The listing builds one solid part. Answer for the finished solid, in the listing's coordinates (mm). A direction names the side the tool comes from. Coordinates: 2 decimals unless noted, no trailing zeros. Loops run counter-clockwise (first coordinate to the right, second up) from the corner with the lowest first, then second, coordinate; pieces in that order, holes last. Notation, with made-up numbers: (39, 23.25) - (64, 23.25) arc R12 ccw to (64, 46.25) - close; hole circle Ø3 at (-9.5, 63). An arc over 180 degrees is marked (long way). Put each result on its own line as item: value.
Autodesk Inventor part; units mm, degrees
ref_plane "YZ Plane" through (0, 0, 0) normal (1, 0, 0) x (0, 1, 0)
ref_plane "XZ Plane" through (0, 0, 0) normal (0, 1, 0) x (-1, 0, 0)
ref_plane "XY Plane" through (0, 0, 0) normal (0, 0, 1) x (1, 0, 0)
sketch "Sketch1" plane through (0, 0, 0) normal (1, 0, 0) x (0, 1, 0)
  line L0 (7, 0.625) -> (0, 0.625)
  line L1 (1, 1.45) -> (1, 3.5)
  line L2 (2, 2.45) -> (2, 1.5)
  line L3 (7, 1.5) -> (7, 0.625)
  line L4 (-1.4, 0) -> (8.4, 0)
  line L5 (1.5, 2.45) -> (2, 2.45)
  line L6 (1, 3.5) -> (1.5, 3.5)
  line L7 (1.5, 3.5) -> (1.5, 2.45)
  line L8 (1, 1.45) -> (0, 1.45)
  line L9 (0, 1.45) -> (0, 0.625)
  line L10 (7, 1.5) -> (2, 1.5)
  point P0 (0, 0)
  dimension "d0" = 7
  dimension "d1" = 0.625
  dimension "d8" = 2.45
  dimension "d10" = 0.5
  dimension "d11" = 0.5
  dimension "d13" = 3.5
  dimension "d16" = 1
  dimension "d31" = 1.45
  dimension "d32" = 1.5
revolve "Revolution1" add sketch "Sketch1" angle 360 about axis through (0, -10, 0) along (0, 1, 0)
sketch "Sketch5" plane through (0, 7, 0) normal (0, 1, 0) x (1, 0, 0)
  circle A0 centre (0, 0) radius 0.75
  dimension "d28" = 1.5
extrude "Extrusion2" cut sketch "Sketch5" against normal blind 3
properties part number "TorsOsc-202511-cell-tower" material "Epoxy Resin"
1) Straight lines are drawn through the part: L1, parallel to X at y = 4.8, z = 0; L2, parallel to Z at x = 2.5, y = 1.25; L3, parallel to X at y = 3.1, z = 0 (3 decimals). For each, find the intervals that lie inside material, in ascending order. Write a range as [from, to].
Found:
L1: x = [-1.5, -0.75], [0.75, 1.5]
L2: z = [-2.45, 2.45]
L3: x = [-1.5, -0.625], [0.625, 1.5]
2) The part is cut by section B-B (z = 0). Give the vertices of the cut face in (x, y) (3 decimals).
Found:
outline: (-3.5, 1) - (-1.45, 1) - (-1.45, 0) - (-0.625, 0) - (-0.625, 4) - (-0.75, 4) - (-0.75, 7) - (-1.5, 7) - (-1.5, 2) - (-2.45, 2) - (-2.45, 1.5) - (-3.5, 1.5) - close; (0.625, 0) - (1.45, 0) - (1.45, 1) - (3.5, 1) - (3.5, 1.5) - (2.45, 1.5) - (2.45, 2) - (1.5, 2) - (1.5, 7) - (0.75, 7) - (0.75, 4) - (0.625, 4) - close
3) Each of these flat-tipped pins is pushed along its axis until it touches: pin 1 (2 mm diameter, centred on x = -1.5, z = 2.5, fed in from -Y); pin 2 (2 mm diameter, centred on x = 0, z = 0, fed in from +Y); pin 3 (1 mm diameter, centred on x = 0, z = 2.5, fed in from +Y); pin 4 (1 mm diameter, centred on x = 0, z = 0, fed in from +Y). Where does it stop, or does it pass through?
Found:
pin 1: stops at y = 1
pin 2: stops at y = 7
pin 3: stops at y = 2
pin 4: passes through
4) The part is cut by section A-A (x = 0). Give the vertices of the cut face in (y, z) (3 decimals), and give its area (4 significant figures).
Found:
outline: (0, -1.45) - (1, -1.45) - (1, -3.5) - (1.5, -3.5) - (1.5, -2.45) - (2, -2.45) - (2, -1.5) - (7, -1.5) - (7, -0.75) - (4, -0.75) - (4, -0.625) - (0, -0.625) - close; (0, 0.625) - (4, 0.625) - (4, 0.75) - (7, 0.75) - (7, 1.5) - (2, 1.5) - (2, 2.45) - (1.5, 2.45) - (1.5, 3.5) - (1, 3.5) - (1, 1.45) - (0, 1.45) - close
area: 14.35 mm^2
5) The part is cut by section D-D (y = 2.5). Give the vertices of the cut face in (x, z) (3 decimals).
Found:
outline: circle Ø3 at (0, 0); hole circle Ø1.25 at (0, 0)
6) The part is cut by section C-C (y = 5). Give the vertices of the cut face in (x, z), and give its area (3 significant figures).
Found:
outline: circle Ø3 at (0, 0); hole circle Ø1.5 at (0, 0)
area: 5.30 mm^2
7) For a pull along X with two mould halves and no side action, classify faces 1 (the face through (-2.4, 1.8, -0.5)), 2 (the face through (0.61, 1.97, -0.14)), 3 (the face through (-2, 2, 0)) as pulls with the +X half, pulls with the -X half, needs draft (parallel to the pull), parting line crosses it, or undercut.
Found:
face 1: parting line crosses it
face 2: undercut
face 3: needs draft
8) For faces 4 (the face through (-2, 1, 0)), 5 (the face through (-2, 1.5, 2)), 6 (the face through (-1.341, 1.254, 3.233)), determine the directions among +Z, -Z, +X, -X, +Y, -Y from which every point of the face is accessible in a straight line to the end or side of a thin tool.
Found:
face 4: -Y
face 5: +Y
face 6: +Y, -Y
